The figure shows three views and two pictorial views of one solid part (mm, origin at its lowest corner). Answer the questions. A direction names the side the tool comes from. Round coordinates to 2 decimals unless told otherwise and drop trailing zeros. Order: outer loops, then holes, each group sorted by start corner. A loop starts at its lowest first (then second) coordinate and runs counter-clockwise, first axis right, second up. Notation, with made-up numbers: (-1, 30) - (12, 30) arc R35 ccw to (12, 68) - close; hole circle Ø3 at (84, -24). An arc over 180 degrees is marked (long way). Use CSV: the item, a comma, the result in double quotes.
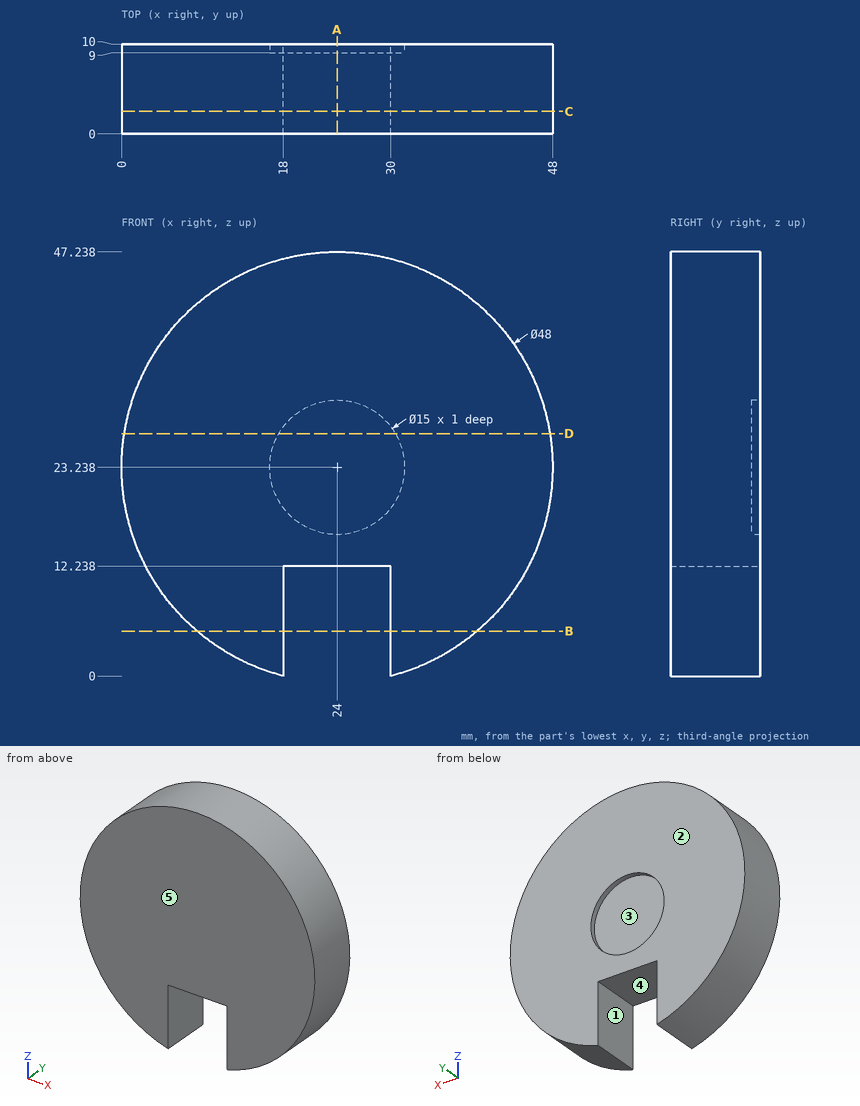
(1) Find section C-C (y = 2.5). Determine the outline of the cut face in (x, z), and give its area (3 significant figures).
Findings below:
outline,"(18, 0) - (18, 12.24) - (30, 12.24) - (30, 0) arc R24 ccw (long way) to start"
area,"1,660 mm²"
(2) Find section D-D (z = 27). Determine the outline of the cut face in (x, y), and give its area (3 significant figures).
Findings below:
outline,"(0.3, 0) - (47.7, 0) - (47.7, 10) - (30.49, 10) - (30.49, 9) - (17.51, 9) - (17.51, 10) - (0.3, 10) - close"
area,"461 mm²"
(3) Each of these flat-tipped pins is pushed along its axis until it touches: pin 1 (6 mm diameter, centred on y = 8, z = 27, fed in from -X); pin 2 (4.5 mm diameter, centred on x = 23.5, z = 25.5, fed in from +Y); pin 3 (5 mm diameter, centred on y = 5.5, z = 4, fed in from +X); pin 4 (2 mm diameter, centred on y = 8, z = 23.5, fed in from +X). Where does it stop, or does it pass through?
Findings below:
pin 1,"stops at x = 0.01"
pin 2,"stops at y = 9"
pin 3,"stops at x = 41.2"
pin 4,"stops at x = 48"
(4) The mould has two halves that part along Z. Classify the marked faces 3, 4 and 5: released by +Z, released by -Z, zero draft, split by the parting line, or undercut.
Findings below:
face 3,"undercut"
face 4,"released by -Z"
face 5,"zero draft"
(5) Find section A-A (x = 24). Determine the outline of the cut face in (y, z).
Findings below:
outline,"(0, 12.24) - (10, 12.24) - (10, 15.74) - (9, 15.74) - (9, 30.74) - (10, 30.74) - (10, 47.24) - (0, 47.24) - close"
(6) Find the intervals of material crossed by L1, parallel to Z at x = 24, y = 9.85; L2, parallel to X at y = 4.5, z = 4.5; L3, parallel to Y at x = 26.5, z = 30, in increasing order. Write a range as from..to.
Findings below:
L1,"z = 12.24..15.74, 30.74..47.24"
L2,"x = 9..18, 30..39"
L3,"y = 0..9"
(7) Find section B-B (z = 5). Determine the outline of the cut face in (x, y), and give its area (3 significant figures).
Findings below:
outline,"(8.4, 0) - (18, 0) - (18, 10) - (8.4, 10) - close; (30, 0) - (39.6, 0) - (39.6, 10) - (30, 10) - close"
area,"192 mm²"
(8) For the marked faces 1 and 2, determine the directions among +Z, -Z, +X, -X, +Y, -Y from which every point of the face is accessible in a straight line to the end or side of a thin tool.
Findings below:
face 1,"-Z, +Y, -Y"
face 2,"+Z, -Z, +X, -X, +Y"
